Design review of the part shown in the three views and the two pictorial views. Dimensions are in mm from the part's minimum x, y and z. Coordinates: 2 decimals unless noted, no trailing zeros. Write each loop counter-clockwise with the first axis right and the second up, starting at its lowest first coordinate (ties: lowest second). Pieces come first, ordered by that corner, then holes. Notation, with made-up numbers: M 22.5,80 L 40.5,80 A6 cw 40.5,85 Z; hole C 13,-9 d3. An arc over 180 degrees is marked long. Answer as a JSON object with one key per item and string values.
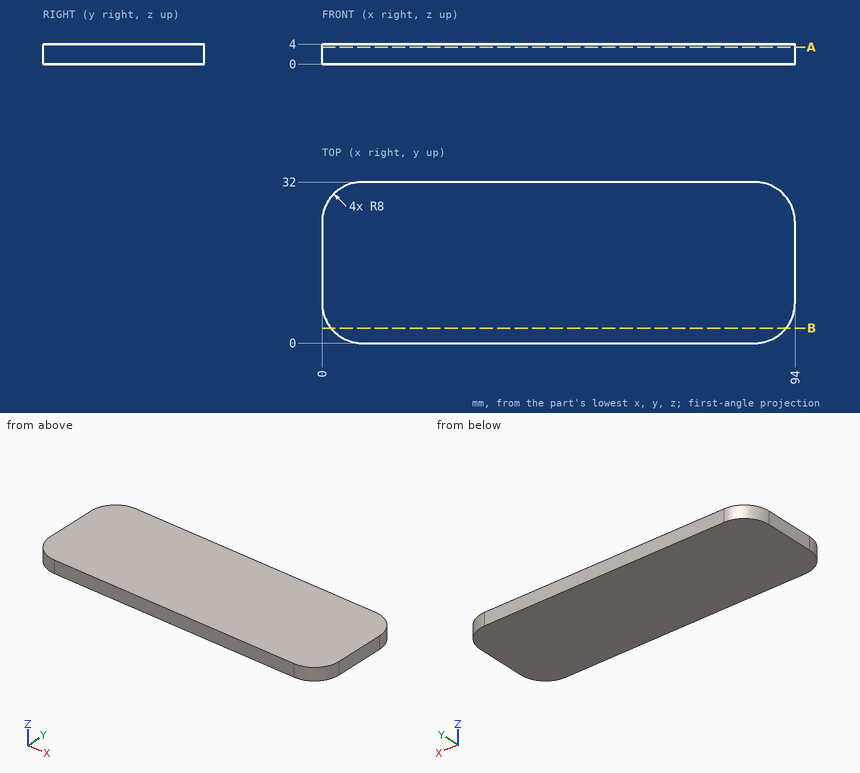
(1) Add section A-A on z = 3.4. Give the boundary of the cut face in (x, y), and give its area (3 significant figures).
Results list:
{"outline": "M 0,8 A8 ccw 8,0 L 86,0 A8 ccw 94,8 L 94,24 A8 ccw 86,32 L 8,32 A8 ccw 0,24 Z", "area": "2,950 mm²"}
(2) Add section B-B on y = 3. Give the boundary of the cut face in (x, z) (3 decimals), and give its area (3 significant figures).
Results list:
{"outline": "M 1.755,0 L 92.245,0 L 92.245,4 L 1.755,4 Z", "area": "362 mm²"}
(3) Wall thickness on line 1 along Y through (x, z) = (6, 2.4); line 2 along X through (y, z) = (5, 2.9); line 3 along X through (y, z) = (26, 3.55): over which ranges is each line inside the solid? List them lowest first. Write a range as from..to.
Results list:
{"line 1": "0.25..31.75", "line 2": "0.58..93.42", "line 3": "0.25..93.75"}
